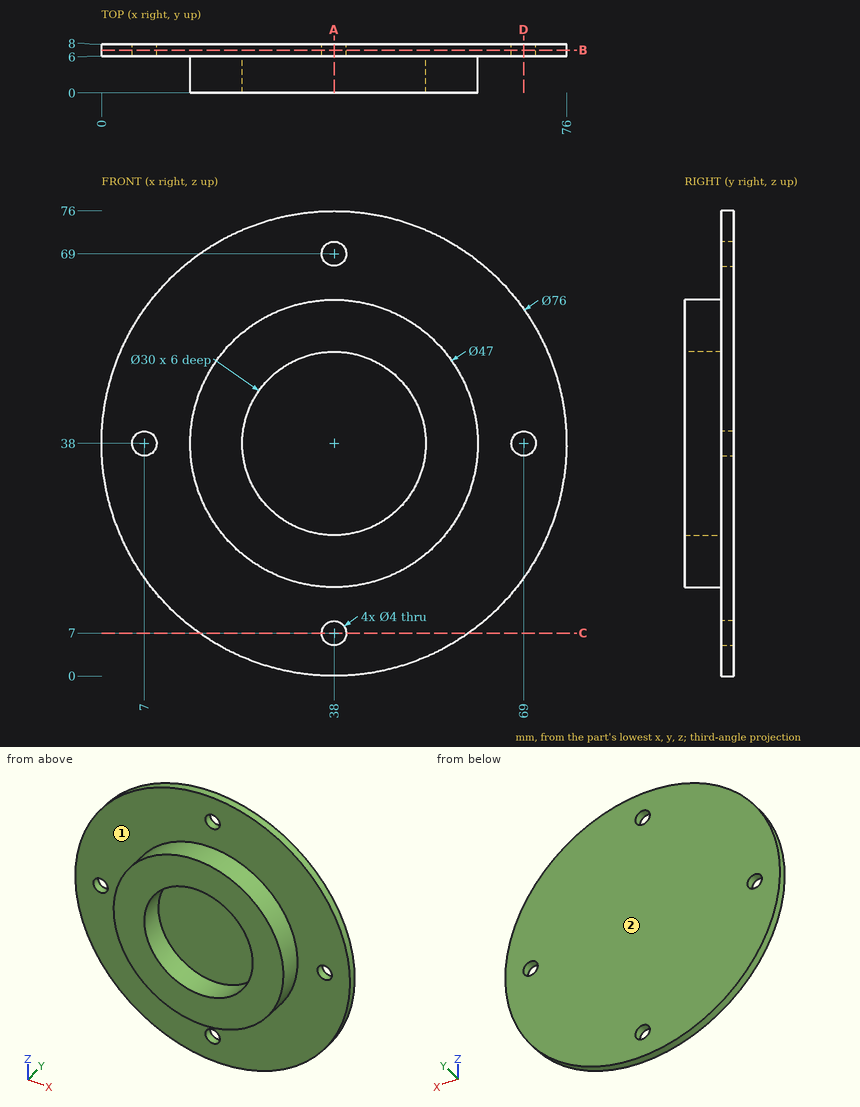
Print and shaded views of the part. All mm, measured from the part's lowest x, y and z. A direction names the side the tool comes from. Round coordinates to 2 decimals unless told otherwise and drop trailing zeros. Order: outer loops, then holes, each group sorted by start corner. A loop starts at its lowest first (then second) coordinate and runs counter-clockwise, first axis right, second up.
Q1. Slice it at D-D (x = 69). Write the cut outline in (y, z), and give its area (3 significant figures).
Q2. Slice it at A-A (x = 38). Write the cut outline in (y, z), and give its area (3 significant figures).
Q3. Slice it at B-B (y = 7). Write the cut outline in (x, z), and give its area (3 significant figures).
Q4. Wall check: L1, parallel to X at y = 7.05, z = 38; L2, parallel to Y at x = 11.5, z = 29; L3, parallel to Z at x = 7, y = 7. Give the ranges that are in metal, low to high.
Q5. Slice it at C-C (z = 7). Write the cut outline in (x, y).
Q6. Drop flat-ended pins along their axis: pin 1 (1.5 mm diameter, centred on x = 58.5, y = 4, fed in from +Z); pin 2 (24 mm diameter, centred on x = 38, z = 38, fed in from -Y); pin 3 (2 mm diameter, centred on x = 26, y = 6.5, fed in from -Z). Give the stop position or say it passes through.
Q7. Which spindle directions (+Z, -Z, +X, -X, +Y, -Y) get a long thin tool onto all of the face, cutting with end or side? Do the marked faces 1 and 2. Say none if no direction does.
Results below:
1. outline: (6, 16.02) - (8, 16.02) - (8, 36) - (6, 36) - close; (6, 40) - (8, 40) - (8, 59.98) - (6, 59.98) - close
1. area: 79.9 mm2
2. outline: (0, 14.5) - (6, 14.5) - (6, 9) - (8, 9) - (8, 67) - (6, 67) - (6, 61.5) - (0, 61.5) - (0, 53) - (6, 53) - (6, 23) - (0, 23) - close; (6, 0) - (8, 0) - (8, 5) - (6, 5) - close; (6, 71) - (8, 71) - (8, 76) - (6, 76) - close
2. area: 238 mm2
3. outline: circle Ø76 at (38, 38); hole circle Ø4 at (7, 38); hole circle Ø4 at (38, 7); hole circle Ø4 at (38, 69); hole circle Ø4 at (69, 38)
3. area: 4,490 mm2
4. L1: x = 0 to 5, 9 to 67, 71 to 76
4. L2: y = 6 to 8
4. L3: z = 16.02 to 36, 40 to 59.98
5. outline: (16.02, 6) - (36, 6) - (36, 8) - (16.02, 8) - close; (40, 6) - (59.98, 6) - (59.98, 8) - (40, 8) - close
6. pin 1: stops at z = 50.74
6. pin 2: stops at y = 6
6. pin 3: stops at z = 1.63
7. face 1: -Y
7. face 2: +Z, -Z, +X, -X, +Y
